Work out the finished part from the listing and answer in its coordinate system (mm). Round coordinates to 2 decimals unless told otherwise and drop trailing zeros. Write each loop counter-clockwise with the first axis right and the second up, starting at its lowest first coordinate (ties: lowest second). Pieces come first, ordered by that corner, then holes. Notation, with made-up numbers: (25, 42.25) - (78, 42.25) arc R13 cw to (78, 56.25) - close; hole circle Ø11 at (43, 11.5). An arc over 180 degrees is marked (long way). Answer as a JSON object with one key per item and string values.
```python
from build123d import *

# Parameters (mm, degrees)
BOSS_EXTRUDE1_DEPTH  = 0.125
SKETCH2_W            = 0.3
SKETCH2_H            = 10
CUT_EXTRUDE1_DEPTH   = 211.481145236
LPATTERN1_COUNT      = 3
LPATTERN1_PITCH      = 20
SKETCH3_W            = 5
SKETCH3_H            = 10
CUT_EXTRUDE2_DEPTH   = 211.481145236
LPATTERN2_COUNT      = 3
LPATTERN2_PITCH      = 20
LPATTERN2_COUNT_DIR2 = 2
LPATTERN2_PITCH_DIR2 = 392


with BuildPart() as part:
    # Sketch1 → Boss-Extrude1 (new, symmetric)
    with BuildSketch(Plane.XY):
        Polygon((0, 0), (193.5, 40), (198.5, 40), (198.5, 70), (193.5, 70), (-193.5, 70), (-198.5, 70), (-198.5, 40), (-193.5, 40), align=None)
    extrude(amount=BOSS_EXTRUDE1_DEPTH, both=True)

    # Sketch2 → Cut-Extrude1 (cut, through all)
    with BuildSketch(Plane.XY.offset(0.125)):
        with Locations((0, 55)):
            Rectangle(SKETCH2_W, SKETCH2_H)
    cut_extrude1 = extrude(amount=-CUT_EXTRUDE1_DEPTH, mode=Mode.SUBTRACT)

    # LPattern1: Cut-Extrude1 ×3
    with Locations(*[(0, -i * LPATTERN1_PITCH, 0) for i in range(1, LPATTERN1_COUNT)]):
        add(cut_extrude1, mode=Mode.SUBTRACT)

    # Sketch3 → Cut-Extrude2 (cut, through all)
    with BuildSketch(Plane.XY.offset(0.125)):
        with Locations((-196, 65)):
            Rectangle(SKETCH3_W, SKETCH3_H)
    cut_extrude2 = extrude(amount=-CUT_EXTRUDE2_DEPTH, mode=Mode.SUBTRACT)

    # LPattern2: Cut-Extrude2 3 × 2
    with Locations(*[(j * LPATTERN2_PITCH_DIR2, -i * LPATTERN2_PITCH, 0) for i in range(LPATTERN2_COUNT) for j in range(LPATTERN2_COUNT_DIR2) if (i, j) != (0, 0)]):
        add(cut_extrude2, mode=Mode.SUBTRACT)


solid = part.part
```
Item 1: Consider line 1 along Y through (x, z) = (0, -0.05); line 2 along X through (y, z) = (41.5, 0.05); line 3 along Y through (x, z) = (139.5, 0.05). Determine where each line is inside the solid, lowest interval first.
Results found:
{"line 1": "0 to 10, 20 to 30, 40 to 50, 60 to 70", "line 2": "-193.5 to 193.5", "line 3": "28.84 to 70"}
Item 2: A cutting plane is placed at C-C (x = -143). Write down the section's boundary in (y, z) (3 decimals), and give its area (3 significant figures).
Results found:
{"outline": "(29.561, -0.125) - (70, -0.125) - (70, 0.125) - (29.561, 0.125) - close", "area": "10.1 mm²"}
Item 3: A cutting plane is placed at B-B (y = 44.5). Write down the section's boundary in (x, z) (3 decimals), and give its area (4 significant figures).
Results found:
{"outline": "(-193.5, -0.125) - (193.5, -0.125) - (193.5, 0.125) - (-193.5, 0.125) - close", "area": "96.75 mm²"}
Item 4: A cutting plane is placed at A-A (z = 0). Write down the section's boundary in (x, y), and give its area (3 significant figures).
Results found:
{"outline": "(-198.5, 50) - (-193.5, 50) - (-193.5, 40) - (0, 0) - (193.5, 40) - (193.5, 50) - (198.5, 50) - (198.5, 60) - (193.5, 60) - (193.5, 70) - (-193.5, 70) - (-193.5, 60) - (-198.5, 60) - close; hole (-0.15, 10) - (0.15, 10) - (0.15, 20) - (-0.15, 20) - close; hole (-0.15, 30) - (0.15, 30) - (0.15, 40) - (-0.15, 40) - close; hole (-0.15, 50) - (0.15, 50) - (0.15, 60) - (-0.15, 60) - close", "area": "19,400 mm²"}
